Here's how the part is built. I have some questions about the finished solid (model axes, mm). Face numbers are marked on the shaded views. A direction names the side the tool comes from. Round coordinates to 2 decimals unless told otherwise and drop trailing zeros. Order: outer loops, then holes, each group sorted by start corner. A loop starts at its lowest first (then second) coordinate and runs counter-clockwise, first axis right, second up. Notation, with made-up numbers: M 84,62 L 141,62 A3 cw 141,66 Z; hole C 40.5,-22.75 d6. An arc over 180 degrees is marked long. Use one line per item in the form item = value. Start each with the question number.
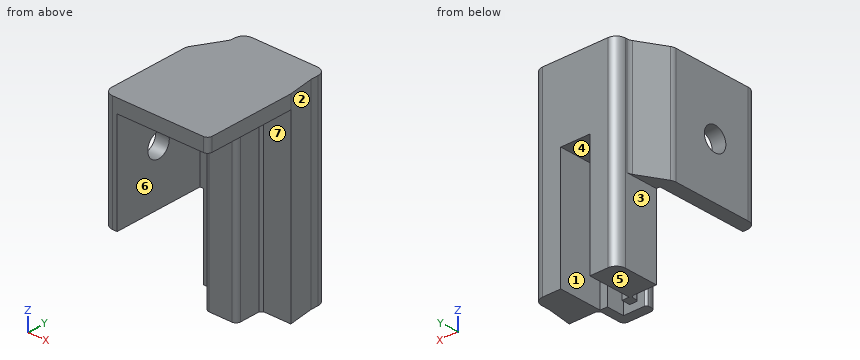
```python
from build123d import *

# Parameters (mm, degrees)
SKETCH_1_W          = 20
SKETCH_1_H          = 20
EXTRUDE_1_DEPTH     = 3
SKETCH_2_W          = 7
SKETCH_2_H          = 6
EXTRUDE_2_DEPTH     = 40
SKETCH_3_W          = 3
SKETCH_3_H          = 20
EXTRUDE_3_DEPTH     = 25
CUT_EXTRUDE_1_REACH = 49.212
SKETCH_4_R          = 2.6
FILLET_1_R          = 1
SKETCH_5_W          = 3.2
SKETCH_5_H          = 3.9
CUT_EXTRUDE_2_DEPTH = 30
SKETCH_6_W          = 6
SKETCH_6_H          = 9.5
EXTRUDE_4_DEPTH     = 43
CHAMFER_1_SIZE      = 0.5
SKETCH_7_W          = 6.4
SKETCH_7_H          = 9.5
EXTRUDE_5_DEPTH     = 16.5
EXTRUDE_6_DEPTH     = 25
FILLET_2_R          = 2
SKETCH_10_W         = 1.9
SKETCH_10_H         = 2
CUT_EXTRUDE_3_DEPTH = 26.5
FILLET_3_R          = 0.5
FILLET_4_R          = 1
EXTRUDE_7_DEPTH     = 43


with BuildPart() as part:
    # ｽｹｯﾁ1 → ﾎﾞｽ - 押し出し1 (new body)
    with BuildSketch(Plane.XY):
        Rectangle(SKETCH_1_W, SKETCH_1_H)
    extrude(amount=EXTRUDE_1_DEPTH)

    # ｽｹｯﾁ2 → ﾎﾞｽ - 押し出し2 (add)
    with BuildSketch(Plane(origin=(0, 0, 0), x_dir=(-1, 0, 0), z_dir=(0, 0, -1))):
        with Locations((0, 7)):
            Rectangle(SKETCH_2_W, SKETCH_2_H)
    extrude(amount=EXTRUDE_2_DEPTH)

    # ｽｹｯﾁ3 → ﾎﾞｽ - 押し出し3 (add)
    with BuildSketch(Plane.XY.offset(3)):
        with Locations((-11.5, 0)):
            Rectangle(SKETCH_3_W, SKETCH_3_H)
    extrude(amount=-EXTRUDE_3_DEPTH)

    # ｽｹｯﾁ4 → ｶｯﾄ - 押し出し1 (cut, up to next)
    with BuildSketch(Plane(origin=(-13, 0, 0), x_dir=(0, 0, -1), z_dir=(1, 0, 0)), mode=Mode.PRIVATE) as cut_extrude_1_sk1:
        with Locations(Location((10, 0, 0), (0, 0, 90))):
            Circle(SKETCH_4_R)
    cut_extrude_1_tool1 = extrude(cut_extrude_1_sk1.sketch, amount=CUT_EXTRUDE_1_REACH, mode=Mode.PRIVATE) & part.part
    add(cut_extrude_1_tool1.solids().sort_by_distance((-13, 0, -10))[0], mode=Mode.SUBTRACT)

    # ﾌｨﾚｯﾄ1
    fillet_1_edges = [part.edges().sort_by_distance(p)[0] for p in [
        (10, -10, 1.5),
    ]]
    fillet(fillet_1_edges, radius=FILLET_1_R)

    # ｽｹｯﾁ5 → ｶｯﾄ - 押し出し2 (cut)
    with BuildSketch(Plane(origin=(0, 0, -13.5), x_dir=(-1, 0, 0), z_dir=(0, 0, -1))):
        with Locations((0, 8.05)):
            Rectangle(SKETCH_5_W, SKETCH_5_H)
    extrude(amount=CUT_EXTRUDE_2_DEPTH, mode=Mode.SUBTRACT)

    # ｽｹｯﾁ6 → ﾎﾞｽ - 押し出し4 (add)
    with BuildSketch(Plane.XY.offset(3)):
        with Locations((6.2, 14.75)):
            Rectangle(SKETCH_6_W, SKETCH_6_H)
        with Locations((-6.2, 14.75)):
            Rectangle(SKETCH_6_W, SKETCH_6_H)
    extrude(amount=-EXTRUDE_4_DEPTH)

    # 面取り1
    chamfer_1_edges = [part.edges().sort_by_distance(p)[0] for p in [
        (-3.5, 10, -20),
        (3.5, 10, -20),
    ]]
    chamfer(chamfer_1_edges, length=CHAMFER_1_SIZE)

    # ｽｹｯﾁ7 → ﾎﾞｽ - 押し出し5 (add)
    with BuildSketch(Plane.XY.offset(3)):
        with Locations((0, 14.75)):
            Rectangle(SKETCH_7_W, SKETCH_7_H)
    extrude(amount=-EXTRUDE_5_DEPTH)

    # ｽｹｯﾁ8 → ﾎﾞｽ - 押し出し6 (add)
    with BuildSketch(Plane.XY.offset(3)):
        Polygon((-13, 10), (-9.2, 10), (-9.2, 16.581793069), align=None)
    extrude(amount=-EXTRUDE_6_DEPTH)

    # ﾌｨﾚｯﾄ2
    fillet_2_edges = [part.edges().sort_by_distance(p)[0] for p in [
        (-9.2, 16.581793069, -9.5),
        (-13, -10, -9.5),
        (-13, 10, -9.5),
        (9.2, 19.5, -18.5),
        (-9.2, 19.5, -18.5),
    ]]
    fillet(fillet_2_edges, radius=FILLET_2_R)

    # ｽｹｯﾁ10 → ｶｯﾄ - 押し出し3 (cut)
    with BuildSketch(Plane(origin=(0, 0, -40), x_dir=(-1, 0, 0), z_dir=(0, 0, -1))):
        with Locations((2.55, 7.1)):
            Rectangle(SKETCH_10_W, SKETCH_10_H)
    extrude(amount=-CUT_EXTRUDE_3_DEPTH, mode=Mode.SUBTRACT)

    # ﾌｨﾚｯﾄ3
    fillet_3_edges = [part.edges().sort_by_distance(p)[0] for p in [
        (-3.5, 6.1, -26.75),
        (-3.5, 8.1, -26.75),
    ]]
    fillet(fillet_3_edges, radius=FILLET_3_R)

    # ﾌｨﾚｯﾄ4
    fillet_4_edges = [part.edges().sort_by_distance(p)[0] for p in [
        (-3.5, 4, -20),
        (3.5, 4, -20),
    ]]
    fillet(fillet_4_edges, radius=FILLET_4_R)

    # ｽｹｯﾁ9 → ﾎﾞｽ - 押し出し7 (add)
    with BuildSketch(Plane.XY.offset(3)):
        Polygon((10, 10), (9.2, 10), (9.2, 15.8), align=None)
    extrude(amount=-EXTRUDE_7_DEPTH)


solid = part.part
```
1) If we section it at D-D on x = 5.5: Write out the boundary of the cut face in (y, z).
2) If we section it at A-A on z = -36.5: Write out the boundary of the cut face in (x, y).
3) If we mould it in two halves opening along X, with no side actions, what happens to the marked faces 1, 2, 3 and 4? For each: +X half, -X half, draft (parallel to the pull), parting line (faces both ways), or undercut.
4) If I drill on line 1 (Z direction, x = -11.75, y = 0); line 2 (X direction, y = 16.75, z = -22.5); line 3 (X direction, y = 5, z = -8.5), over which ranges is the centre line in solid material (lowest first)?
5) If we section it at B-B on y = 0: Write out the boundary of the cut face in (x, z), then the cut area to 3 significant figures.
6) On a 3-axis mill with a long thin cutter (end or side, diameter ignored), from which of +Z, -Z, +X, -X, +Y, -Y can I reach the whole of each face in a straight line? I mean the marked faces 5, 6 and 7. Say none if no direction works.
7) Will these pins go through, and if not, where does the flat tip stop? pin 1 Ø5 at (x, z) = (1.5, -28) entering from -Y; pin 2 Ø1.3 at (y, z) = (7, -12.5) entering from +X; pin 3 Ø3 at (x, y) = (-10.5, 8.5) entering from -Z.
8) If we section it at C-C on z = -10: Write out the boundary of the cut face in (x, y).
Completed:
q1.outline = M -10,0 L 10,0 L 10,-40 L 19.5,-40 L 19.5,3 L -10,3 Z
q2.outline = M -9.2,10 L -4,10 L -3.5,9.5 L -3.5,8.6 A0.5 ccw -3,8.1 L -1.6,8.1 L -1.6,10 L -3.2,10 L -3.2,19.5 L -7.2,19.5 A2 ccw -9.2,17.5 Z; M -3.5,5 A1 ccw -2.5,4 L 2.5,4 A1 ccw 3.5,5 L 3.5,9.5 L 4,10 L 10,10 L 9.2,15.8 L 9.2,17.5 A2 ccw 7.2,19.5 L 3.2,19.5 L 3.2,10 L 1.6,10 L 1.6,6.1 L -3,6.1 A0.5 ccw -3.5,5.6 Z
q3.face_1 = undercut
q3.face_2 = +X half
q3.face_3 = -X half
q3.face_4 = undercut
q4.line_1 = -22 to -12.6, -7.4 to 3
q4.line_2 = -9.2 to -3.2, 3.2 to 9.2
q4.line_3 = -13 to -10, -3.5 to 3.5
q5.outline = M -13,-22 L -10,-22 L -10,-12.6 L -13,-12.6 Z; M -13,-7.4 L -10,-7.4 L -10,0 L 10,0 L 10,3 L -13,3 Z
q5.area = 119 mm²
q6.face_5 = -Z, +X, -X, +Y, -Y
q6.face_6 = -Z, -Y
q6.face_7 = -Z, +X, -Y
q7.pin_1 = 4
q7.pin_2 = 3.5
q7.pin_3 = -22
q8.outline = M -13,-8 A2 ccw -11,-10 L -10,-10 L -10,-2.6 L -13,-2.6 Z; M -13,2.6 L -10,2.6 L -10,10 L -4,10 L -3.5,9.5 L -3.5,5 A1 ccw -2.5,4 L 2.5,4 A1 ccw 3.5,5 L 3.5,9.5 L 4,10 L 10,10 L 9.2,15.8 L 9.2,17.5 A2 ccw 7.2,19.5 L -7.2,19.5 A2 ccw -9.2,17.5 L -9.2,17.12 A2 cw -9.47,16.12 L -12.73,10.46 A2 ccw -13,9.46 Z
